The figure shows three views and two pictorial views of one solid part (mm, origin at its lowest corner). Answer the questions. Give positions to 0.01 mm unless a question says otherwise; leave off trailing zeros. Order: outer loops, then holes, each group sorted by start corner. A loop starts at its lowest first (then second) coordinate and runs counter-clockwise, first axis right, second up. Notation, with made-up numbers: (-6.75, 47) - (50.25, 47) arc R4 ccw to (50.25, 54) - close; hole circle Ø2 at (13, -0.75). An arc over 180 degrees is marked (long way). Write item = value, one per line.
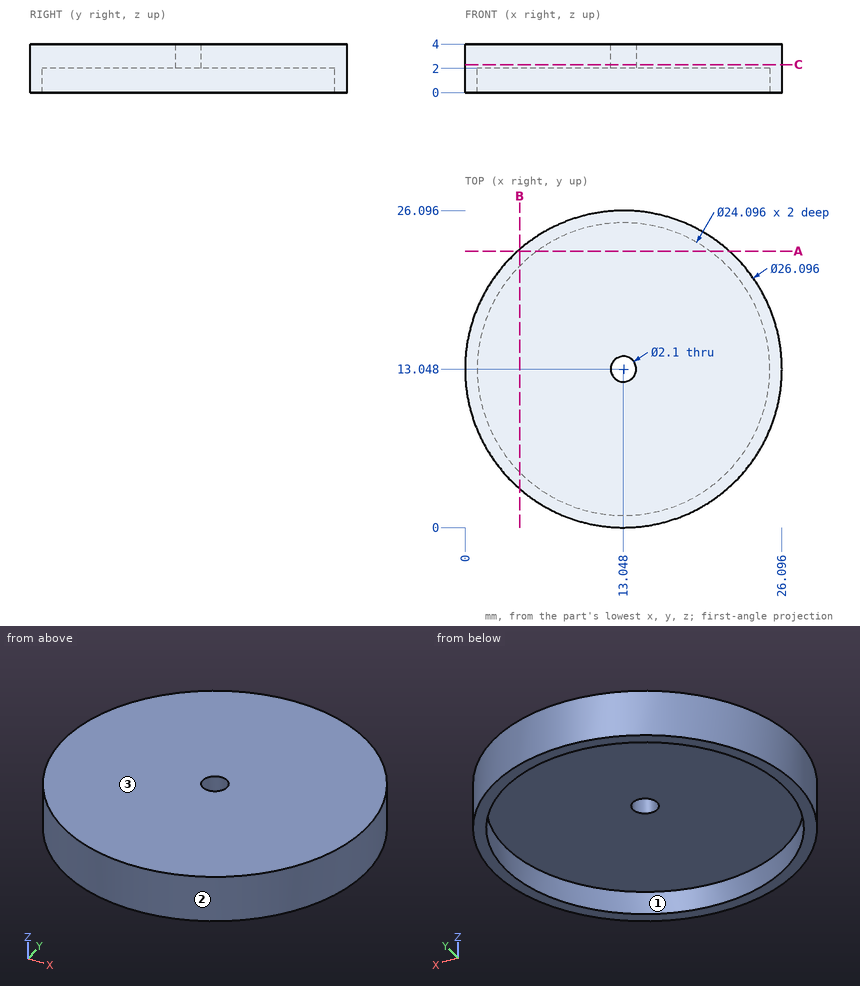
1. Straight lines are drawn through the part: L1, parallel to Z at x = 18.75, y = 3.25; L2, parallel to X at y = 7, z = 1.6 (1 decimal); L3, parallel to X at y = 13, z = 2.75. For each, find the intervals that lie inside material, in ascending order. Write a range as [from, to].
Recorded:
L1 = [2, 4]
L2 = [1.5, 2.6], [23.5, 24.6]
L3 = [0, 12], [14.1, 26.1]
2. Section A-A (y = 22.75) is taken. Determine the outline of the cut face in (x, z) (1 decimal).
Recorded:
outline = (4.3, 0) - (5.9, 0) - (5.9, 2) - (20.2, 2) - (20.2, 0) - (21.8, 0) - (21.8, 4) - (4.3, 4) - close
3. Section C-C (z = 2.3) is taken. Determine the outline of the cut face in (x, y), and give its area (3 significant figures).
Recorded:
outline = circle Ø26.1 at (13.05, 13.05); hole circle Ø2.1 at (13.05, 13.05)
area = 531 mm^2
4. Flat-ended cylindrical pins translate along their axes: pin 1 (3 mm diameter, centred on x = 16, y = 19.5, fed in from -Z); pin 2 (14.5 mm diameter, centred on x = 13.05, y = 13.05, fed in from +Z); pin 3 (2 mm diameter, centred on y = 18.5, z = 0.5, fed in from -X); pin 4 (1.7 mm diameter, centred on x = 13.05, y = 13.05, fed in from -Z). Find the tip coordinate at first contact, or state that the pin passes through.
Recorded:
pin_1 = 2
pin_2 = 4
pin_3 = 0.78
pin_4 = through
5. Section B-B (x = 4.5) is taken. Determine the outline of the cut face in (y, z), and give its area (3 significant figures).
Recorded:
outline = (3.19, 0) - (4.56, 0) - (4.56, 2) - (21.54, 2) - (21.54, 0) - (22.91, 0) - (22.91, 4) - (3.19, 4) - close
area = 44.9 mm^2
6. Determine the mould class of the marked faces 1, 2 and 3 for opening direction X: +X half, -X half, draft (parallel to the pull), parting line (faces both ways), or undercut.
Recorded:
face_1 = undercut
face_2 = parting line
face_3 = draft
